Source: three-view drawing plus pictorial views. Frame: mm from the lowest corner of the part. A direction names the side the tool comes from. Coordinates: 2 decimals unless noted, no trailing zeros. Loops run counter-clockwise (first coordinate to the right, second up) from the corner with the lowest first, then second, coordinate; pieces in that order, holes last. Notation, with made-up numbers: (11, -3.5) - (29, -3.5) arc R9 ccw to (29, 0.5) - close; hole circle Ø5 at (67.25, 76). An arc over 180 degrees is marked (long way). Use CSV: the item, a comma, the result in double quotes. Start each with the question number.
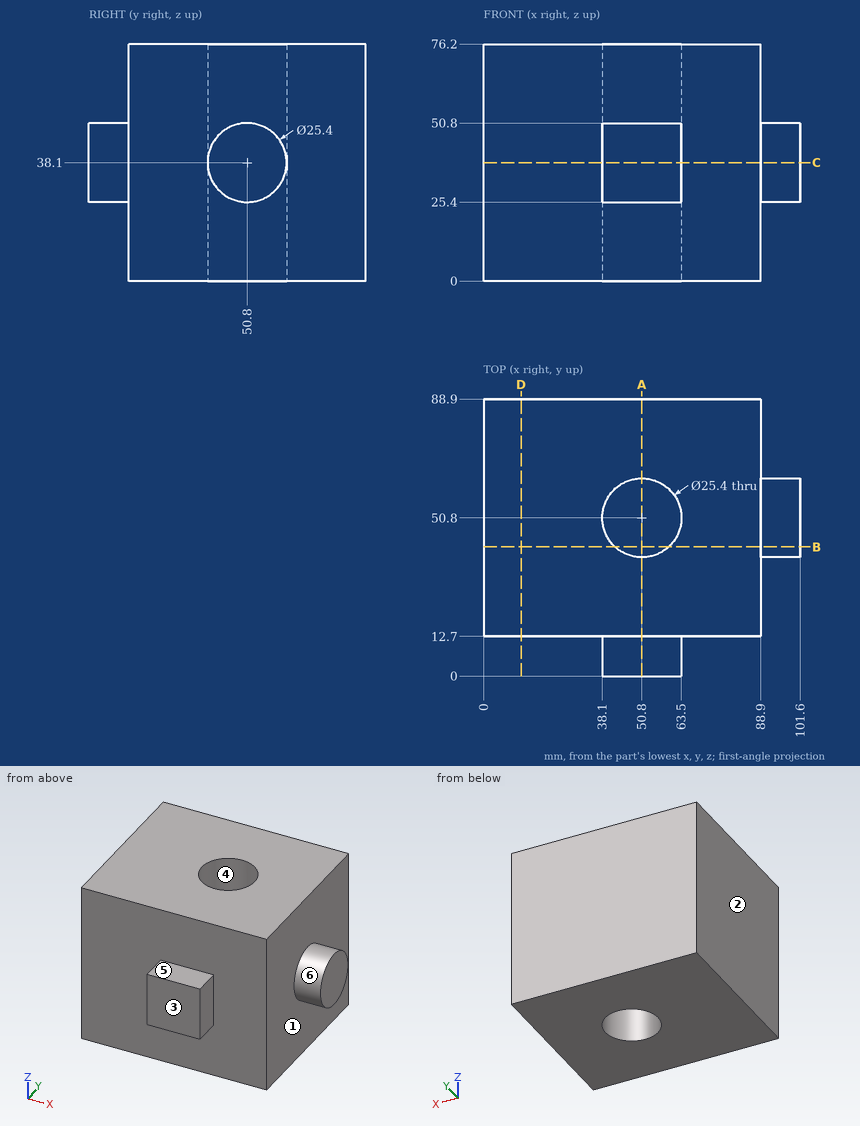
(1) Draft query along Y for the marked faces 3, 4, 5 and 6. Return one class per face: released by +Y, released by -Y, zero draft, split by the parting line, or undercut.
(2) Section C-C on z = 38.1. Output: boundary loops of the cut face in (x, y).
(3) Section D-D on x = 12. Output: boundary loops of the cut face in (y, z).
(4) Reachability of the marked faces 1 and 2 from +Z, -Z, +X, -X, +Y, -Y: full face, straight path, thin tool, end or side. Return the list, or none.
(5) Ray query, line 1 (Y direction, x = 50, z = 24); line 2 (Y direction, x = 65, z = 30.5); line 3 (X direction, y = 50, z = 48). Return the intervals inside material, ascending. Write a range as [from, to].
(6) Section A-A on x = 50.8. Output: boundary loops of the cut face in (y, z), plus the area to 3 significant figures.
(7) Pin query (flat end, axial travel): pin 1 Ø14 at (y, z) = (6.5, 35.5) entering from +X; pin 2 Ø1.5 at (x, z) = (81.5, 25) entering from -Y; pin 3 Ø6.5 at (y, z) = (5.5, 38) entering from -X. Return the tip coordinate at first contact, or that it passes through.
(8) Section B-B on y = 41.5. Output: boundary loops of the cut face in (x, z).
Solution:
1,face 3,"released by -Y"
1,face 4,"undercut"
1,face 5,"zero draft"
1,face 6,"split by the parting line"
2,outline,"(0, 12.7) - (38.1, 12.7) - (38.1, 0) - (63.5, 0) - (63.5, 12.7) - (88.9, 12.7) - (88.9, 38.1) - (101.6, 38.1) - (101.6, 63.5) - (88.9, 63.5) - (88.9, 88.9) - (0, 88.9) - close; hole circle Ø25.4 at (50.8, 50.8)"
3,outline,"(12.7, 0) - (88.9, 0) - (88.9, 76.2) - (12.7, 76.2) - close"
4,face 1,"+X"
4,face 2,"+Z, -Z, -X, +Y, -Y"
5,line 1,"y = [12.7, 38.13], [63.47, 88.9]"
5,line 2,"y = [12.7, 88.9]"
5,line 3,"x = [0, 38.13], [63.47, 101.6]"
6,outline,"(0, 25.4) - (12.7, 25.4) - (12.7, 0) - (38.1, 0) - (38.1, 76.2) - (12.7, 76.2) - (12.7, 50.8) - (0, 50.8) - close; (63.5, 0) - (88.9, 0) - (88.9, 76.2) - (63.5, 76.2) - close"
6,area,"4,190 mm²"
7,pin 1,"stops at x = 88.9"
7,pin 2,"stops at y = 12.7"
7,pin 3,"stops at x = 38.1"
8,outline,"(0, 0) - (42.15, 0) - (42.15, 76.2) - (0, 76.2) - close; (59.45, 0) - (88.9, 0) - (88.9, 29.45) - (101.6, 29.45) - (101.6, 46.75) - (88.9, 46.75) - (88.9, 76.2) - (59.45, 76.2) - close"
